from build123d import *

# Parameters (mm, degrees)
F0_R         = 11
F1_DEPTH     = 7
F2_T1_DEPTH  = 53.4348218988
F2_T3_DEPTH  = 53.3566125342
F2_T5_DEPTH  = 53.6604130231
F2_T7_DEPTH  = 53.7564599562
F2_T9_DEPTH  = 54.3050348939
F2_T11_DEPTH = 54.0874720662
F3_T1_DEPTH  = 53.4348218988
F3_T3_DEPTH  = 53.6604130231
F3_T5_DEPTH  = 53.7564599562
F3_T7_DEPTH  = 54.3050348939
F3_T9_DEPTH  = 54.0874720662
F3_T11_DEPTH = 53.3566125342


# Not quite as in the source:
# - a fillet or chamfer that OpenCascade refuses, or shapes differently, is made with other operations: its cross-section is extruded or revolved along the edge and cut away or added


with BuildPart() as f1:
    # F0 (on Top) → F1 (new body)
    with BuildSketch(Plane.XY):
        with BuildLine():
            Line((19.2151323873, 22.3788071315), (0, 55.077418685))
            Line((0, 55.077418685), (-19.066227053, 22.2013174855))
            ThreePointArc((-19.066227053, 22.2013174855), (-15.2197508504, 8.7138440156), (-28.8366321548, 5.35410246))
            Line((-28.8366321548, 5.35410246), (-48.0160338648, -27.7171470225))
            Line((-48.0160338648, -27.7171470225), (-9.6896718364, -27.7171470225))
            ThreePointArc((-9.6896718364, -27.7171470225), (0.0445471902, -17.5375945189), (9.7787662169, -27.7171470225))
            Line((9.7787662169, -27.7171470225), (48.6537031829, -27.7171470225))
            Line((48.6537031829, -27.7171470225), (29.0682872932, 5.6115802214))
            ThreePointArc((29.0682872932, 5.6115802214), (15.2034219667, 8.7426653076), (19.2151323873, 22.3788071315))
        make_face()
        with Locations((-24.3902284877, -14.0817042541)):
            Circle(F0_R, mode=Mode.SUBTRACT)
        Circle(F0_R, mode=Mode.SUBTRACT)
        with Locations((24.3902285123, -14.0817042399)):
            Circle(F0_R, mode=Mode.SUBTRACT)
        with Locations((0, 28.1634107232)):
            Circle(F0_R, mode=Mode.SUBTRACT)
    extrude(amount=F1_DEPTH)

    # F2: chamfer of 3 on 6 edges, made by hand

    # F2_s2 → F2_t1 (cut)
    with BuildSketch(Plane(origin=(27.7729977796, 47.8892799857, 0), x_dir=(0, 0, 1), z_dir=(-0.5016804508, -0.8650530188, 0))):
        Polygon((4, 27.6312642329), (7, 24.6312642329), (7, 27.6312642329), align=None)
    extrude(amount=F2_T1_DEPTH, mode=Mode.SUBTRACT)

    # F2_s4 → F2_t3 (cut)
    with BuildSketch(Plane(origin=(-0.9341553956, 1.5896629696, 0), x_dir=(0, 0, 1), z_dir=(-0.5066411345, 0.8621570396, 0))):
        Polygon((4, 27.9044858871), (7, 24.9044858871), (7, 27.9044858871), align=None)
    extrude(amount=F2_T3_DEPTH, mode=Mode.SUBTRACT)

    # F2_s6 → F2_t5 (cut)
    with BuildSketch(Plane(origin=(-1.0636343753, -1.8340362392, 0), x_dir=(0, 0, 1), z_dir=(-0.5016804508, -0.8650530188, 0))):
        Polygon((4, 27.6312642329), (7, 24.6312642329), (7, 27.6312642329), align=None)
    extrude(amount=F2_T5_DEPTH, mode=Mode.SUBTRACT)

    # F2_s8 → F2_t7 (cut)
    with BuildSketch(Plane.YZ.offset(-55.7310828287)):
        Polygon((-27.7171470225, 4), (-24.7171470225, 7), (-27.7171470225, 7), align=None)
    extrude(amount=F2_T7_DEPTH, mode=Mode.SUBTRACT)

    # F2_s10 → F2_t9 (cut)
    with BuildSketch(Plane.YZ.offset(2.063717253)):
        Polygon((-27.7171470225, 4), (-24.7171470225, 7), (-27.7171470225, 7), align=None)
    extrude(amount=F2_T9_DEPTH, mode=Mode.SUBTRACT)

    # F2_s12 → F2_t11 (cut)
    with BuildSketch(Plane(origin=(28.5044154, -48.5062911843, 0), x_dir=(0, 0, 1), z_dir=(-0.5066411345, 0.8621570396, 0))):
        Polygon((4, 27.9044858871), (7, 24.9044858871), (7, 27.9044858871), align=None)
    extrude(amount=F2_T11_DEPTH, mode=Mode.SUBTRACT)

    # F3: chamfer of 3 on 6 edges, made by hand

    # F3_s2 → F3_t1 (cut)
    with BuildSketch(Plane(origin=(27.7729977796, 47.8892799857, 0), x_dir=(0, 0, 1), z_dir=(-0.5016804508, -0.8650530188, 0))):
        Polygon((0, 24.6312642329), (3, 27.6312642329), (0, 27.6312642329), align=None)
    extrude(amount=F3_T1_DEPTH, mode=Mode.SUBTRACT)

    # F3_s4 → F3_t3 (cut)
    with BuildSketch(Plane(origin=(-1.0636343753, -1.8340362392, 0), x_dir=(0, 0, 1), z_dir=(-0.5016804508, -0.8650530188, 0))):
        Polygon((0, 24.6312642329), (3, 27.6312642329), (0, 27.6312642329), align=None)
    extrude(amount=F3_T3_DEPTH, mode=Mode.SUBTRACT)

    # F3_s6 → F3_t5 (cut)
    with BuildSketch(Plane.YZ.offset(-55.7310828287)):
        Polygon((-24.7171470225, 0), (-27.7171470225, 3), (-27.7171470225, 0), align=None)
    extrude(amount=F3_T5_DEPTH, mode=Mode.SUBTRACT)

    # F3_s8 → F3_t7 (cut)
    with BuildSketch(Plane.YZ.offset(2.063717253)):
        Polygon((-24.7171470225, 0), (-27.7171470225, 3), (-27.7171470225, 0), align=None)
    extrude(amount=F3_T7_DEPTH, mode=Mode.SUBTRACT)

    # F3_s10 → F3_t9 (cut)
    with BuildSketch(Plane(origin=(28.5044154, -48.5062911843, 0), x_dir=(0, 0, 1), z_dir=(-0.5066411345, 0.8621570396, 0))):
        Polygon((0, 24.9044858871), (3, 27.9044858871), (0, 27.9044858871), align=None)
    extrude(amount=F3_T9_DEPTH, mode=Mode.SUBTRACT)

    # F3_s12 → F3_t11 (cut)
    with BuildSketch(Plane(origin=(-0.9341553956, 1.5896629696, 0), x_dir=(0, 0, 1), z_dir=(-0.5066411345, 0.8621570396, 0))):
        Polygon((0, 24.9044858871), (3, 27.9044858871), (0, 27.9044858871), align=None)
    extrude(amount=F3_T11_DEPTH, mode=Mode.SUBTRACT)


solid = f1.part
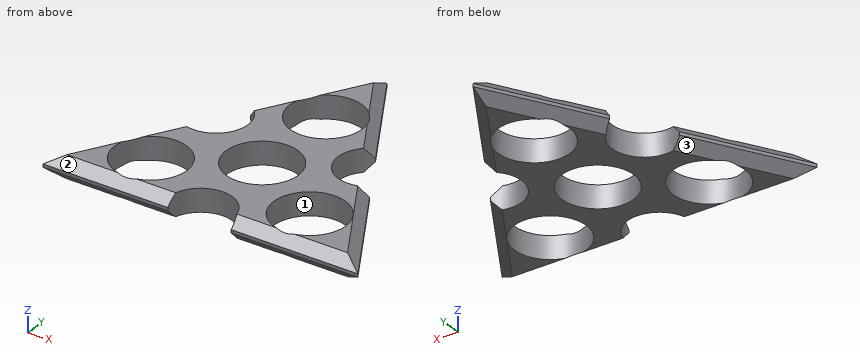
Source: CAD feature listing. Evaluate the final solid. Frame: model axes, mm. Face numbers are marked on the shaded views. Coordinates: 2 decimals unless noted, no trailing zeros. Loops run counter-clockwise (first coordinate to the right, second up) from the corner with the lowest first, then second, coordinate; pieces in that order, holes last. Notation, with made-up numbers: (-8, 67.25) - (37, 67.25) arc R33 cw to (37, 98.25) - close; hole circle Ø9 at (52.25, 76.25). An arc over 180 degrees is marked (long way). One line per question, with ' | ' between items.
1) Section C-C, the plane z = 1.75. Return loops of the section in (x, y).
Report:
outline: (-45.85, -26.47) - (-9.67, -26.47) arc R9.74 cw to (9.75, -26.47) - (46.47, -26.47) - (27.99, 4.98) arc R9.74 cw to (18.14, 21.75) - (0.01, 52.6) - (-18, 21.54) arc R9.74 cw to (-27.74, 4.76) - close; hole circle Ø22 at (-24.39, -14.08); hole circle Ø22 at (0, 0); hole circle Ø22 at (0, 28.16); hole circle Ø22 at (24.39, -14.08)
2) Section A-A, the plane x = 32. Return loops of the section in (y, z).
Report:
outline: (-27.72, 3) - (-24.72, 0) - (-22.02, 0) - (-22.02, 7) - (-24.72, 7) - (-27.72, 4) - close; (-6.14, 0) - (-5.3, 0) - (0.62, 3) - (0.62, 4) - (-5.3, 7) - (-6.14, 7) - close
3) Line query: line 1 along Y through (x, z) = (-10, 3); line 2 along Y through (x, z) = (-1.5, 1.25); line 3 along X through (y, z) = (-21, 3.75). Output: solid intervals per line, ascending.
Report:
line 1: y = -27.72 to -4.58, 4.58 to 23.58, 32.75 to 37.83 | line 2: y = -17.66 to -10.9, 10.9 to 17.27, 39.06 to 49 | line 3: x = -44.12 to -32.94, -15.84 to -7.4, 7.49 to 15.84, 32.94 to 44.71
4) Section B-B, the plane y = 27. Return loops of the section in (x, z).
Report:
outline: (-16.28, 3) - (-12.82, 0) - (-10.94, 0) - (-10.94, 7) - (-12.82, 7) - (-16.28, 4) - close; (10.94, 0) - (13.02, 0) - (16.5, 3) - (16.5, 4) - (13.02, 7) - (10.94, 7) - close
5) First-contact query: P1, Ø1.5, axis at x = 27, z = 5.5, coming from the -Y side; P2, Ø2, axis at y = 32.5, z = 4, coming from the +X side; P3, Ø1.5, axis at y = -16.5, z = 2, coming from the +X side. Flat tips, straight axial feed; report the tip coordinate or a pass-through.
Report:
P1: stops at y = -26.97 | P2: stops at x = 13.86 | P3: stops at x = 41.88
6) Pull-direction query (X, two-part tool) for the marked faces 1, 2 and 3; classes: released by +X, released by -X, zero draft, split by the parting line, or undercut.
Report:
face 1: undercut | face 2: zero draft | face 3: released by -X
7) Section D-D, the plane y = -8. Give the number of separate pieces and of enclosed holes in the cut face, then the cut area to 3 significant figures.
Report:
separate pieces: 4 | enclosed holes: 0 | area: 133 mm²
